For this review, take the finished solid that the model builds, in its own axes (mm). A direction names the side the tool comes from. Coordinates: 2 decimals unless noted, no trailing zeros. Write each loop counter-clockwise with the first axis right and the second up, starting at its lowest first coordinate (ties: lowest second). Pieces come first, ordered by that corner, then holes. Notation, with made-up numbers: M 29.25,-8 L 77.25,-8 A24 ccw 77.25,29 Z; hole C 74,80 d8. An arc over 180 degrees is marked long. One line per question, with ' | ' between items.
from build123d import *

# Parameters (mm, degrees)
F0_R          = 3.1
F1_DEPTH      = 35
F2_R          = 2
F3_DEPTH      = 31.501
F3_DEPTH_BACK = 0.301
F5_DEPTH      = 25.901


# Not quite as in the source:
# - a feature names something its author has since deleted; it is built from what else it names


with BuildPart() as f1:
    # F0 (on Top) → F1 (new body)
    with BuildSketch(Plane.XY):
        with BuildLine():
            ThreePointArc((-27.9, 0), (-26.7577164466, -2.7577164466), (-24, -3.9))
            ThreePointArc((-24, -3.9), (-21.2422835534, -2.7577164466), (-20.1, 0))
            ThreePointArc((-20.1, 0), (-21.2422835534, 2.7577164466), (-24, 3.9))
            ThreePointArc((-24, 3.9), (-26.643179735, 2.8676821456), (-27.8870765814, 0.3172312247))
            Line((-27.8870765814, 0.3172312247), (-27.9, 0))
        make_face()
        with Locations((-24, 0)):
            Circle(F0_R, mode=Mode.SUBTRACT)
        with BuildLine():
            Line((-27.6, 7.3641016151), (-27.8870765814, 0.3172312247))
            ThreePointArc((-27.8870765814, 0.3172312247), (-26.643179735, 2.8676821456), (-24, 3.9))
            ThreePointArc((-24, 3.9), (-25.4641016151, 5.3641016151), (-26, 7.3641016151))
            Line((-26, 7.3641016151), (-26, 22))
            Line((-26, 22), (-27.6, 22))
            Line((-27.6, 22), (-27.6, 7.3641016151))
        make_face()
        with BuildLine():
            ThreePointArc((0, -3.9), (-2.7577164466, -2.7577164466), (-3.9, 0))
            Line((-3.9, 0), (-3.9, 0.1))
            ThreePointArc((-3.9, 0.1), (-4.4857864376, -1.3142135624), (-5.9, -1.9))
            Line((-5.9, -1.9), (-18.1, -1.9))
            ThreePointArc((-18.1, -1.9), (-19.5142135624, -1.3142135624), (-20.1, 0.1))
            Line((-20.1, 0.1), (-20.1, 0))
            ThreePointArc((-20.1, 0), (-21.2422835534, -2.7577164466), (-24, -3.9))
            Line((-24, -3.9), (0, -3.9))
        make_face()
        with BuildLine():
            Line((3.9, 0), (3.8870765814, 0.3172312247))
            ThreePointArc((3.8870765814, 0.3172312247), (2.643179735, 2.8676821456), (0, 3.9))
            ThreePointArc((0, 3.9), (-2.7577164466, 2.7577164466), (-3.9, 0))
            ThreePointArc((-3.9, 0), (-2.7577164466, -2.7577164466), (0, -3.9))
            ThreePointArc((0, -3.9), (2.7577164466, -2.7577164466), (3.9, 0))
        make_face()
        Circle(F0_R, mode=Mode.SUBTRACT)
        with BuildLine():
            Line((3.6, 7.3641016151), (3.6, 22))
            Line((3.6, 22), (2, 22))
            Line((2, 22), (2, 7.3641016151))
            ThreePointArc((2, 7.3641016151), (1.4641016151, 5.3641016151), (0, 3.9))
            ThreePointArc((0, 3.9), (2.643179735, 2.8676821456), (3.8870765814, 0.3172312247))
            Line((3.8870765814, 0.3172312247), (3.6, 7.3641016151))
        make_face()
    extrude(amount=F1_DEPTH)

    # F2 (on face) → F3 (cut, two sides)
    with BuildSketch(Plane.YZ.offset(3.6)) as f3_sk:
        with BuildLine():
            ThreePointArc((18.5, 21.5), (20.9748737342, 20.4748737342), (22, 18))
            Line((22, 18), (22, 35))
            Line((22, 35), (7.3641016151, 35))
            Line((7.3641016151, 35), (7.3641016151, 24.4293139302))
            Line((7.3641016151, 24.4293139302), (10.1173140978, 22.8397459622))
            ThreePointArc((10.1173140978, 22.8397459622), (12.5291236468, 21.8407417371), (15.1173140978, 21.5))
            Line((15.1173140978, 21.5), (18.5, 21.5))
        make_face()
        Polygon((22, 35), (22, 18), (29.6666024476, 18), (29.6666024476, 42.8468726724), (-4.3945980379, 42.8468726724), (-4.3945980379, 31.2182023401), (7.3641016151, 24.4293139302), (7.3641016151, 35), align=None)
        with Locations((18.5, 18)):
            Circle(F2_R)
        with BuildLine():
            Line((22, 0), (22, 18))
            ThreePointArc((22, 18), (21.7007350945, 16.5839156612), (20.8541172259, 15.4099938057))
            Line((20.8541172259, 15.4099938057), (7.3641016151, 3.1486030042))
            Line((7.3641016151, 3.1486030042), (7.3641016151, 0))
            Line((7.3641016151, 0), (22, 0))
        make_face()
        Polygon((7.3641016151, 0), (7.3641016151, 3.1486030042), (3.9, 0), align=None)
    extrude(amount=-F3_DEPTH, mode=Mode.SUBTRACT)
    extrude(f3_sk.sketch, amount=F3_DEPTH_BACK, mode=Mode.SUBTRACT)

    # F4 (on face) → F5 (cut, through all)
    with BuildSketch(Plane.XZ.offset(3.9)):
        with BuildLine():
            ThreePointArc((-12, 0), (-6.3431457505, 2.3431457505), (-4, 8))
            ThreePointArc((-4, 8), (-12, 16), (-20, 8))
            ThreePointArc((-20, 8), (-17.6568542495, 2.3431457505), (-12, 0))
        make_face()
        with BuildLine():
            Line((-4, 0), (-4, 8))
            ThreePointArc((-4, 8), (-6.3431457505, 2.3431457505), (-12, 0))
            Line((-12, 0), (-4, 0))
        make_face()
        with BuildLine():
            ThreePointArc((-12, 0), (-17.6568542495, 2.3431457505), (-20, 8))
            Line((-20, 8), (-20, 0))
            Line((-20, 0), (-12, 0))
        make_face()
        with BuildLine():
            Line((0, 30.9326460298), (0, 26.4293139302))
            Line((0, 26.4293139302), (8.4664272144, 26.4293139302))
            Line((8.4664272144, 26.4293139302), (8.4664272144, 34.5878303051))
            Line((8.4664272144, 34.5878303051), (-3.2313269012, 34.5878303051))
            ThreePointArc((-3.2313269012, 34.5878303051), (-2.6846257606, 32.7964600712), (-2.5, 30.9326460298))
            Line((-2.5, 30.9326460298), (0, 30.9326460298))
        make_face()
        with BuildLine():
            Line((-3.6351927697, 26.4293139302), (0, 26.4293139302))
            Line((0, 26.4293139302), (0, 30.9326460298))
            Line((0, 30.9326460298), (-2.5, 30.9326460298))
            ThreePointArc((-2.5, 30.9326460298), (-2.7881687844, 28.6105423164), (-3.6351927697, 26.4293139302))
        make_face()
        with BuildLine():
            Line((-24, 30.9326460298), (-24, 26.4293139302))
            Line((-24, 26.4293139302), (-20.3648072303, 26.4293139302))
            ThreePointArc((-20.3648072303, 26.4293139302), (-21.2118312156, 28.6105423164), (-21.5, 30.9326460298))
            Line((-21.5, 30.9326460298), (-24, 30.9326460298))
        make_face()
        with BuildLine():
            Line((-31.3403680921, 26.4293139302), (-24, 26.4293139302))
            Line((-24, 26.4293139302), (-24, 30.9326460298))
            Line((-24, 30.9326460298), (-21.5, 30.9326460298))
            ThreePointArc((-21.5, 30.9326460298), (-21.3153742394, 32.7964600712), (-20.7686730988, 34.5878303051))
            Line((-20.7686730988, 34.5878303051), (-31.3403680921, 34.5878303051))
            Line((-31.3403680921, 34.5878303051), (-31.3403680921, 26.4293139302))
        make_face()
        with BuildLine():
            Line((-20.3648072303, 26.4293139302), (-3.6351927697, 26.4293139302))
            ThreePointArc((-3.6351927697, 26.4293139302), (-2.7881687844, 28.6105423164), (-2.5, 30.9326460298))
            Line((-2.5, 30.9326460298), (-21.5, 30.9326460298))
            ThreePointArc((-21.5, 30.9326460298), (-21.2118312156, 28.6105423164), (-20.3648072303, 26.4293139302))
        make_face()
        with BuildLine():
            ThreePointArc((-20.3648072303, 26.4293139302), (-12, 21.4326460298), (-3.6351927697, 26.4293139302))
            Line((-3.6351927697, 26.4293139302), (-20.3648072303, 26.4293139302))
        make_face()
    extrude(amount=-F5_DEPTH, mode=Mode.SUBTRACT)


solid = f1.part
1) Machinability: for faces 4 (the flat face through (-4, -2, 4)), 5 (the cylindrical face through (-27, 12, 22)), 6 (the flat face through (-26, 13, 16)), 7 (the flat face through (3.6, 13, 16)), 8 (the cylindrical face through (1.43, -2.75, 13.03)), which of the approach directions +Z, -Z, +X, -X, +Y, -Y give a long, thin tool a straight path to every point of the face, cutting with its end or side? Answer none if there is none.
Responses:
face 4: -Z, +Y, -Y | face 5: +Z, +X, -X, +Y | face 6: +Z, -Z, +Y | face 7: +Z, -Z, +X, +Y | face 8: +Z, -Z
2) To check wall thickness, follow line 1 along Y through (x, z) = (-24, 8.75); line 2 along X through (y, z) = (1.5, 1.25); line 3 along X through (y, z) = (17, 14.75). State the ranges of each line that lie inside material, in increasing order. Write a range as [from, to].
Responses:
line 1: [-3.9, -3.1], [3.1, 3.9] | line 2: [-27.84, -26.71], [-21.29, -20.4], [-3.6, -2.71], [2.71, 3.84] | line 3: [-27.6, -26], [2, 3.6]
3) We need section D-D on y = -1.25. State the section outline as (x, z) points, then the cut area to 3 significant figures.
Responses:
outline: M -27.69,0 L -26.84,0 L -26.84,26.43 L -27.69,26.43 Z; M -21.16,0 L -20,0 L -20,8 A8 cw -19.58,10.57 L -19.58,25.2 A9.5 cw -20.36,26.43 L -21.16,26.43 Z; M -4.42,10.57 A8 cw -4,8 L -4,0 L -2.84,0 L -2.84,26.43 L -3.64,26.43 A9.5 cw -4.42,25.2 Z; M 2.84,0 L 3.69,0 L 3.69,26.43 L 2.84,26.43 Z | area: 120 mm^2
4) We need section B-B on y = 14.5. State the section outline as (x, z) points, then the cut area to 3 significant figures.
Responses:
outline: M -27.6,9.63 L -26,9.63 L -26,21.52 L -27.6,21.52 Z; M 2,9.63 L 3.6,9.63 L 3.6,21.52 L 2,21.52 Z | area: 38.0 mm^2
5) The part is to be moulded in two halves that separate along Z. For faces 1 (the flat face through (-27, 17, 21.5)), 2 (the flat face through (-15, -3.9, 16)), 3 (the cylindrical face through (2.811, 18.24, 19.983)), say which applies: +Z half, -Z half, draft (parallel to the pull), parting line (faces both ways), or undercut.
Responses:
face 1: +Z half | face 2: draft | face 3: undercut
6) We need section A-A on z = 18.75. State how many separate pieces and enclosed holes the cut face has, then the cut area to 3 significant figures.
Responses:
separate pieces: 3 | enclosed holes: 2 | area: 132 mm^2
7) We need section C-C on x = -22.5. State the section outline as (y, z) points, then the cut area to 3 significant figures.
Responses:
outline: M -3.9,0 L -2.71,0 L -2.71,26.43 L -3.9,26.43 Z; M 2.71,0 L 3.6,0 L 3.6,26.43 L 2.71,26.43 Z | area: 54.8 mm^2
8) Insertion check: pin 1 Ø6.5 at (y, z) = (18.5, 18) entering from +X; pin 2 Ø2.5 at (y, z) = (-2.5, 5) entering from -X; pin 3 Ø7.5 at (y, z) = (15.5, 13.5) entering from -X. Each pin has a flat end and moves straight along its axis. Give the tip position at first contact, or say it passes through.
Responses:
pin 1: x = 3.6 | pin 2: x = -27.69 | pin 3: x = -27.6
